Check sheet for the modelled part. Datum: model origin and axes. Units: mm. A direction names the side the tool comes from. Round coordinates to 2 decimals unless told otherwise and drop trailing zeros. Order: outer loops, then holes, each group sorted by start corner. A loop starts at its lowest first (then second) coordinate and runs counter-clockwise, first axis right, second up.
```python
from build123d import *

# Parameters (mm, degrees)
F0_W      = 30
F0_H      = 5
F1_DEPTH  = 150
F2_W      = 95
F2_H      = 5
F3_DEPTH  = 30
F4_W      = 10
F4_H      = 5
F5_DEPTH  = 120
F7_DEPTH  = 5
F8_W      = 65
F8_H      = 5
F9_DEPTH  = 50
F11_DEPTH = 5
F12_W     = 95
F12_H     = 10
F13_DEPTH = 10
F14_W     = 5.5
F14_H     = 30
F15_DEPTH = 2
F16_W     = 4
F16_H     = 30
F17_DEPTH = 3
F18_W     = 8
F18_H     = 10
F19_DEPTH = 1


with BuildPart() as f1:
    # F0 (on Top) → F1 (new body)
    with BuildSketch(Plane.XY):
        Polygon((0, 20), (0, 0), (10, 0), (10, 15), (10, 20), align=None)
        with Locations((25, 17.5)):
            Rectangle(F0_W, F0_H)
    extrude(amount=F1_DEPTH)

    # F2 (on Top) → F3 (join)
    with BuildSketch(Plane.XY):
        with Locations((57.5, 2.5)):
            Rectangle(F2_W, F2_H)
    extrude(amount=F3_DEPTH)

    # F4 (on face) → F5 (join)
    with BuildSketch(Plane.XY.offset(30)):
        with Locations((15, 2.5)):
            Rectangle(F4_W, F4_H)
    extrude(amount=F5_DEPTH)

    # F6 (on face) → F7 (join)
    with BuildSketch(Plane.XZ):
        Polygon((30, 30), (20, 150), (20, 30), align=None)
    extrude(amount=-F7_DEPTH)

    # F8 (on Top) → F9 (join)
    with BuildSketch(Plane.XY):
        with Locations((72.5, 17.5)):
            Rectangle(F8_W, F8_H)
    extrude(amount=F9_DEPTH)

    # F10 (on face) → F11 (join)
    with BuildSketch(Plane(origin=(0, 20, 0), x_dir=(-1, 0, 0), z_dir=(0, 1, 0))):
        Polygon((-90, 50), (-40, 50), (-40, 150), align=None)
    extrude(amount=-F11_DEPTH)

    # F12 (on Top) → F13 (join)
    with BuildSketch(Plane.XY):
        with Locations((57.5, 10)):
            Rectangle(F12_W, F12_H)
    extrude(amount=F13_DEPTH)

    # F14 (on face) → F15 (join)
    with BuildSketch(Plane.XZ):
        with Locations((107.75, 15)):
            Rectangle(F14_W, F14_H)
    extrude(amount=-F15_DEPTH)

    # F16 (on face) → F17 (join)
    with BuildSketch(Plane.XZ):
        with Locations((112.5, 15)):
            Rectangle(F16_W, F16_H)
    extrude(amount=-F17_DEPTH)

    # F18 (on face) → F19 (cut)
    with BuildSketch(Plane(origin=(0, 0, 0), x_dir=(0, -1, 0), z_dir=(-1, 0, 0))):
        with Locations((-10, 35)):
            Rectangle(F18_W, F18_H)
        with Locations((-10, 85)):
            Rectangle(F18_W, F18_H)
        with Locations((-10, 135)):
            Rectangle(F18_W, F18_H)
    extrude(amount=-F19_DEPTH, mode=Mode.SUBTRACT)


solid = f1.part
```
Item 1: Go/stop test with flat-tipped pins: P1, Ø12, axis at y = 8, z = 96.5, coming from the +X side; P2, Ø12, axis at x = 102.5, y = 13.5, coming from the +Z side; P3, Ø10, axis at x = 92, z = 58, coming from the +Y side; P4, Ø1.6, axis at x = 109, z = 18.5, coming from the +Y side. Record where each tip stops, or that it passes through.
Answer:
P1: stops at x = 24.89
P2: stops at z = 50
P3: passes through
P4: stops at y = 2
Item 2: Access from +Z, -Z, +X, -X, +Y, -Y to the whole of each face (thin tool, end or side, straight path). Record for faces 4 (the flat face through (48, 15, 65)), 5 (the flat face through (97, 18, 50)), 6 (the flat face through (1, 10, 135)), 7 (the flat face through (25.07, 2.46, 89.16)).
Answer:
face 4: +Z, +X
face 5: +Z, +X, +Y, -Y
face 6: -X
face 7: +Z, +X, -Y
Item 3: Sectioned sample at B-B (y = 7.75). Record the cut outline in (x, z), and give its area (3 significant figures).
Answer:
outline: (0, 0) - (105, 0) - (105, 10) - (10, 10) - (10, 150) - (0, 150) - (0, 140) - (1, 140) - (1, 130) - (0, 130) - (0, 90) - (1, 90) - (1, 80) - (0, 80) - (0, 40) - (1, 40) - (1, 30) - (0, 30) - close
area: 2,420 mm2
Item 4: Release check for a two-part mould opening along Y. For faces 1 (the flat face through (0, 10, 74)), 2 (the flat face through (26, 5, 54)), 3 (the flat face through (18, 0, 43)) record: released by +Y, released by -Y, zero draft, split by the parting line, or undercut.
Answer:
face 1: zero draft
face 2: undercut
face 3: released by -Y
Item 5: Sectioned sample at D-D (x = 34.5). Record the cut outline in (y, z), and give its area (3 significant figures).
Answer:
outline: (0, 0) - (20, 0) - (20, 150) - (15, 150) - (15, 10) - (5, 10) - (5, 30) - (0, 30) - close
area: 1,000 mm2
Item 6: Sectioned sample at A-A (x = 46). Record the cut outline in (y, z).
Answer:
outline: (0, 0) - (20, 0) - (20, 138) - (15, 138) - (15, 10) - (5, 10) - (5, 30) - (0, 30) - close
Item 7: Scan lines: line 1 along Y through (x, z) = (11, 53); line 2 along Y through (x, z) = (47.5, 55.5); line 3 along Z through (x, y) = (80.5, 3). Record each from-to range of solid material in increasing order.
Answer:
line 1: y = 0 to 5, 15 to 20
line 2: y = 15 to 20
line 3: z = 0 to 30
Item 8: Sectioned sample at C-C (z = 13.5). Record the cut outline in (x, y), and give its area (3 significant figures).
Answer:
outline: (0, 0) - (114.5, 0) - (114.5, 3) - (110.5, 3) - (110.5, 2) - (105, 2) - (105, 5) - (10, 5) - (10, 15) - (105, 15) - (105, 20) - (0, 20) - close
area: 1,170 mm2
